Input: part model. Units: mm. Frame: model coordinates. A direction names the side the tool comes from. Coordinates: 2 decimals unless noted, no trailing zeros. Write each loop counter-clockwise with the first axis right and the second up, starting at its lowest first coordinate (ties: lowest second). Pieces come first, ordered by that corner, then holes. Notation, with made-up numbers: M 76.5,74 L 96.5,74 A28 ccw 96.5,110 Z; hole C -13,26 d9. An arc over 180 degrees is marked long. Write each question's results on one line, items separated by ' | '. Start each with the question number.
1. Ray query, probe 1 along Y at (x, z) = (-1.5, 2.6); probe 2 along X at (y, z) = (2.5, 2.4); probe 3 along X at (y, z) = (2, 2.4). Return the intervals inside material, ascending.
2. First-contact query: pin 1 (0.9 mm diameter, centred on y = 1.5, z = 1.5, fed in from +X); pin 2 (1 mm diameter, centred on y = 8, z = 2.5, fed in from +X). Flat tips, straight axial feed; report the tip coordinate or a pass-through.
3. Section query D-D, the plane x = 5.5. Output: boundary loops of the cut face in (y, z).
4. Section query C-C, the plane z = 1.6. Output: boundary loops of the cut face in (x, y) (1 decimal), and give its area (3 significant figures).
5. Section query A-A, the plane y = 0. Output: boundary loops of the cut face in (x, z) (1 decimal), and give its area (3 significant figures).
6. Pull-direction query (X, two-part tool) for faces 3 (the flat face through (-4.636, 0, 1)), 4 (the cylindrical face through (7.956, -7.296, 1.421)), 5 (the flat face through (-5, 0, 0)); classes: +X half, -X half, draft (parallel to the pull), parting line (faces both ways), or undercut.
7. Set-up query: faces 1 (the flat face through (-5, 0, 2.883)), 2 (the flat face through (0, -4.636, 1)). Return all of +Z, -Z, +X, -X, +Y, -Y with unobstructed straight access to the full face (end or side cutting, diameter ignored); none if empty.
```python
from build123d import *

# Parameters (mm, degrees)
SKETCH1_R           = 10.795
SKETCH1_W           = 9.271
SKETCH1_H           = 9.271
BOSS_EXTRUDE1_DEPTH = 2.8829


with BuildPart() as part:
    # Sketch1 → Boss-Extrude1 (new body)
    with BuildSketch(Plane.XY):
        with Locations(Location((0, 0, 0), (0, 0, 180))):
            Circle(SKETCH1_R)
        Rectangle(SKETCH1_W, SKETCH1_H, mode=Mode.SUBTRACT)
    extrude(amount=BOSS_EXTRUDE1_DEPTH)


solid = part.part
```
Answer:
1) probe 1: -10.69 to -4.64, 4.64 to 10.69 | probe 2: -10.5 to -4.64, 4.64 to 10.5 | probe 3: -10.61 to -4.64, 4.64 to 10.61
2) pin 1: x = 10.74 | pin 2: x = 7.76
3) outline: M -9.29,0 L 9.29,0 L 9.29,2.88 L -9.29,2.88 Z
4) outline: C 0,0 d21.6; hole M -4.6,-4.6 L 4.6,-4.6 L 4.6,4.6 L -4.6,4.6 Z | area: 280 mm^2
5) outline: M -10.8,0 L -4.6,0 L -4.6,2.9 L -10.8,2.9 Z; M 4.6,0 L 10.8,0 L 10.8,2.9 L 4.6,2.9 Z | area: 35.5 mm^2
6) face 3: undercut | face 4: parting line | face 5: draft
7) face 1: +Z, +X, -X, +Y, -Y | face 2: +Z, -Z
